```python
from build123d import *

# Parameters (mm, degrees)
F0_W     = 285.75
F0_H     = 66.675
F1_DEPTH = 508
F2_W     = 285.75
F2_H     = 66.675
F2_W_2   = 228.6
F2_H_2   = 47.625
F3_DEPTH = 66.675
F4_R     = 89.296875
F4_W     = 143.51
F4_H     = 44.45
F5_DEPTH = 66.676


with BuildPart() as f1:
    # F0 (on Front) → F1 (new body)
    with BuildSketch(Plane.XZ):
        Rectangle(F0_W, F0_H)
    extrude(amount=F1_DEPTH)

    # F2 (on face) → F3 (cut)
    with BuildSketch(Plane.XZ.offset(508)):
        Rectangle(F2_W, F2_H)
        Rectangle(F2_W_2, F2_H_2, mode=Mode.SUBTRACT)
    extrude(amount=-F3_DEPTH, mode=Mode.SUBTRACT)

    # F4 (on face) → F5 (cut, through all)
    with BuildSketch(Plane.XY.offset(33.3375)):
        with Locations((0, -276.82825)):
            Circle(F4_R)
        with BuildLine():
            Line((71.755, -44.45), (-71.755, -44.45))
            ThreePointArc((-71.755, -44.45), (0, -116.205), (71.755, -44.45))
        make_face()
        with Locations((0, -22.225)):
            Rectangle(F4_W, F4_H)
    extrude(amount=-F5_DEPTH, mode=Mode.SUBTRACT)


solid = f1.part
```
Could you check a few things on this model? Use its own coordinates, in mm. A direction names the side the tool comes from. Coordinates: 2 decimals unless noted, no trailing zeros. Order: outer loops, then holes, each group sorted by start corner. A loop starts at its lowest first (then second) coordinate and runs counter-clockwise, first axis right, second up. Notation, with made-up numbers: M 9.5,36 L 14.5,36 A17 ccw 14.5,58 Z; hole C -38.5,-32 d6. An arc over 180 degrees is marked long. Use a Markdown table: item, result. Add a question column.
Q1. I want a section at C-C on z = -6.5. List the corners of the cut face in (x, y) for me (3 decimals), then the cut area to 3 significant figures.
Q2. I'm going to push flat-ended pins straight in: pin 1 (1.5 mm diameter, centred on x = 38.5, z = 3, fed in from +Y); pin 2 (20 mm diameter, centred on x = -18.5, y = -486, fed in from +Z); pin 3 (14.5 mm diameter, centred on y = -473, z = 5.5, fed in from +X). Where does each tip first touch, or does it pass through?
Q3. I want a section at D-D on x = 97.5. List the corners of the cut face in (y, z) for me (1 decimal), then the cut area to 3 significant figures.
Q4. I want a section at B-B on y = -246.5. List the corners of the cut face in (x, z) for me (1 decimal), then the cut area to 3 significant figures.
Q5. If I drill on L1, parallel to Y at x = 0, z = -6 (3 decimals); L2, parallel to Y at x = 121, z = -28 (3 decimals); L3, parallel to Y at x = 66, z = 25.5 (1 decimal), over which ranges is the centre line in solid material (lowest first)?
Q6. I want a section at A-A on x = 0. List the corners of the cut face in (y, z) for me (1 decimal), then the cut area to 3 significant figures.
Q7. Which directions (+Z, -Z, +X, -X, +Y, -Y) give clear straight access to the entire face, cutting with the end or side of a thin tool? Please do faces 5 (the flat face through (-114.3, -475, 0)), 6 (the flat face through (-2, -508, 0)), 7 (the flat face through (-2, -475, -23.812)), 8 (the flat face through (-2, -475, 23.812)), 9 (the flat face through (-71.755, -23, 0)).
Q8. We'd pull the mould along X, two halves only. Please class faces 1 (the flat face through (114.3, -475, 0)), 2 (the flat face through (-2, -169, -33.338)), 3 (the flat face through (-142.875, -218, 0)), 4 (the flat face through (71.755, -23, 0)): pulls with the +X half, pulls with the -X half, needs draft (parallel to the pull), parting line crosses it, or undercut.
Checked values:
| question | item | result |
|---|---|---|
| 1 | outline | M -142.875,-441.325 L -114.3,-441.325 L -114.3,-508 L 114.3,-508 L 114.3,-441.325 L 142.875,-441.325 L 142.875,0 L 71.755,0 L 71.755,-44.45 A71.755 cw -71.755,-44.45 L -71.755,0 L -142.875,0 Z; hole C 0,-276.828 d178.594 |
| 1 | area | 102,000 mm² |
| 2 | pin 1 | y = -104.52 |
| 2 | pin 2 | z = 23.81 |
| 2 | pin 3 | x = 114.3 |
| 3 | outline | M -508,-23.8 L -441.3,-23.8 L -441.3,-33.3 L 0,-33.3 L 0,33.3 L -441.3,33.3 L -441.3,23.8 L -508,23.8 Z |
| 3 | area | 32,600 mm² |
| 4 | outline | M -142.9,-33.3 L -84,-33.3 L -84,33.3 L -142.9,33.3 Z; M 84,-33.3 L 142.9,-33.3 L 142.9,33.3 L 84,33.3 Z |
| 4 | area | 7,850 mm² |
| 5 | L1 | -508 to -366.125, -187.531 to -116.205 |
| 5 | L2 | -441.325 to 0 |
| 5 | L3 | -441.3 to -337, -216.7 to -72.6 |
| 6 | outline | M -508,-23.8 L -441.3,-23.8 L -441.3,-33.3 L -366.1,-33.3 L -366.1,33.3 L -441.3,33.3 L -441.3,23.8 L -508,23.8 Z; M -187.5,-33.3 L -116.2,-33.3 L -116.2,33.3 L -187.5,33.3 Z |
| 6 | area | 12,900 mm² |
| 7 | face 5 | +Z, -Z, -X, -Y |
| 7 | face 6 | +Z, -Z, +X, -X, -Y |
| 7 | face 7 | -Z, +X, -X, -Y |
| 7 | face 8 | +Z, +X, -X, -Y |
| 7 | face 9 | +Z, -Z, +Y |
| 8 | face 1 | pulls with the +X half |
| 8 | face 2 | needs draft |
| 8 | face 3 | pulls with the -X half |
| 8 | face 4 | undercut |
